CAD build for the part. Positions are in the model's coordinates, mm. Face numbers are marked on the shaded views. A direction names the side the tool comes from. Give positions to 0.01 mm unless a question says otherwise; leave off trailing zeros. Order: outer loops, then holes, each group sorted by start corner. A loop starts at its lowest first (then second) coordinate and runs counter-clockwise, first axis right, second up. Notation, with made-up numbers: (1.5, 12.5) -> (29.5, 12.5) arc R27 ccw to (29.5, 45.5) -> close; hole circle Ø8 at (50, 87.25). An arc over 180 degrees is marked (long way). Use one line per item in the form item = value. Start each with the question number.
1) Cut at B-B, the plane y = 15. Give the cut face in (x, z) (3 decimals), and give its area (3 significant figures).
2) Mould opens along Z. For the marked faces 4 and 5 say: pulls with the +Z half, pulls with the -Z half, needs draft (parallel to the pull), parting line crosses it, or undercut.
3) Cut at C-C, the plane z = -52. Give the cut face in (x, y) (3 decimals).
4) Cut at A-A, the plane x = 13.75. Give the cut face in (y, z) (3 decimals), and give its area (3 significant figures).
5) Drop flat-ended pins along their axis: P1, Ø12.5, axis at y = 14, z = -52, coming from the +X side; P2, Ø0.8, axis at x = 7, y = 41, coming from the +Z side (3 decimals); P3, Ø9, axis at y = -35, z = -30, coming from the +X side. Give the stop position or say it passes through.
6) Probe line 1 (Z direction, x = 6, y = 43) (3 decimals); line 2 (Z direction, x = 7.25, y = -13) (3 decimals); line 3 (Z direction, x = 6.5, y = -43) (3 decimals). List the from-to ranges inside material, lowest first.
7) Tool access for the marked faces 1, 2 and 3: list every direction of +Z, -Z, +X, -X, +Y, -Y with a clear straight run to the whole face (end or side of a thin tool).
8) Cut at D-D, the plane y = -39. Give the cut face in (x, z) (3 decimals).
from build123d import *

# Parameters (mm, degrees)
SKETCH1_W            = 100
SKETCH1_H            = 130
SKETCH1_W_2          = 32.89
SKETCH1_H_2          = 100.13
SKETCH1_R            = 1
BOSS_EXTRUDE1_DEPTH  = 5
SKETCH3_W            = 32.89
SKETCH3_H            = 100.13
SKETCH3_R            = 1
BOSS_EXTRUDE3_DEPTH  = 3
SKETCH4_W            = 16.6
SKETCH4_H            = 21.6
BOSS_EXTRUDE4_DEPTH  = 2.5
SKETCH5_W            = 60
SKETCH5_H            = 25
BOSS_EXTRUDE5_DEPTH  = 2.5
SKETCH6_W            = 18
SKETCH6_H            = 21
BOSS_EXTRUDE6_DEPTH  = 2
SKETCH7_W            = 8.4
SKETCH7_H            = 20
BOSS_EXTRUDE7_DEPTH  = 5
SKETCH9_W            = 2.5
SKETCH9_H            = 64.8
BOSS_EXTRUDE8_DEPTH  = 5
SKETCH10_W           = 23.22
SKETCH10_H           = 2.5
BOSS_EXTRUDE9_DEPTH  = 18.22
SKETCH12_W           = 26
SKETCH12_H           = 36
BOSS_EXTRUDE11_DEPTH = 5
SKETCH11_W           = 26
SKETCH11_H           = 36
BOSS_EXTRUDE10_DEPTH = 5


with BuildPart() as part:
    # Sketch1 → Boss-Extrude1 (new body)
    # profile 1 of 2: a face of its own
    with BuildSketch(Plane(origin=(0, 0, 0), x_dir=(0, 0, -1), z_dir=(1, 0, 0))):
        with Locations((32.555, -9.935)):
            Rectangle(SKETCH1_W, SKETCH1_H)
        Rectangle(SKETCH1_W_2, SKETCH1_H_2, mode=Mode.SUBTRACT)
    # profile 2 of 2: a face of its own
    with BuildSketch(Plane(origin=(0, 0, 0), x_dir=(0, 0, -1), z_dir=(1, 0, 0))):
        Rectangle(SKETCH1_W_2, SKETCH1_H_2)
        with Locations((-13.855, -47.705)):
            Circle(SKETCH1_R, mode=Mode.SUBTRACT)
        with Locations((13.855, -47.705)):
            Circle(SKETCH1_R, mode=Mode.SUBTRACT)
        with Locations((13.855, 47.395)):
            Circle(SKETCH1_R, mode=Mode.SUBTRACT)
        with Locations((-13.855, 47.395)):
            Circle(SKETCH1_R, mode=Mode.SUBTRACT)
    extrude(amount=BOSS_EXTRUDE1_DEPTH)

    # Sketch3 → Boss-Extrude3 (add)
    with BuildSketch(Plane(origin=(5, 0, 0), x_dir=(0, 0, -1), z_dir=(1, 0, 0))):
        Rectangle(SKETCH3_W, SKETCH3_H)
        with Locations((-13.855, 47.395)):
            Circle(SKETCH3_R, mode=Mode.SUBTRACT)
        with Locations((13.855, 47.395)):
            Circle(SKETCH3_R, mode=Mode.SUBTRACT)
        with Locations((13.855, -47.705)):
            Circle(SKETCH3_R, mode=Mode.SUBTRACT)
        with Locations((-13.855, -47.705)):
            Circle(SKETCH3_R, mode=Mode.SUBTRACT)
    extrude(amount=BOSS_EXTRUDE3_DEPTH)

    # Sketch4 → Boss-Extrude4 (add)
    with BuildSketch(Plane(origin=(5, 0, 0), x_dir=(0, 0, -1), z_dir=(1, 0, 0))):
        with Locations((27.245, 39.265)):
            Rectangle(SKETCH4_W, SKETCH4_H)
    extrude(amount=BOSS_EXTRUDE4_DEPTH)

    # Sketch5 → Boss-Extrude5 (add)
    with BuildSketch(Plane(origin=(5, 0, 0), x_dir=(0, 0, -1), z_dir=(1, 0, 0))):
        with Locations((48.445, 13.965)):
            Rectangle(SKETCH5_W, SKETCH5_H)
    extrude(amount=BOSS_EXTRUDE5_DEPTH)

    # Sketch6 → Boss-Extrude6 (add)
    with BuildSketch(Plane(origin=(5, 0, 0), x_dir=(0, 0, -1), z_dir=(1, 0, 0))):
        with Locations((47.260487744, 39.246233232)):
            Rectangle(SKETCH6_W, SKETCH6_H)
    extrude(amount=BOSS_EXTRUDE6_DEPTH)

    # Sketch7 → Boss-Extrude7 (add)
    with BuildSketch(Plane(origin=(5, 0, 0), x_dir=(0, 0, -1), z_dir=(1, 0, 0))):
        with Locations((62.460487744, 38.465)):
            Rectangle(SKETCH7_W, SKETCH7_H)
    extrude(amount=BOSS_EXTRUDE7_DEPTH)

    # Sketch9 → Boss-Extrude8 (add)
    with BuildSketch(Plane(origin=(5, 0, 0), x_dir=(0, 0, -1), z_dir=(1, 0, 0))):
        with Locations((20.195, -35.935)):
            Rectangle(SKETCH9_W, SKETCH9_H)
        with Locations((40.915, -35.935)):
            Rectangle(SKETCH9_W, SKETCH9_H)
    extrude(amount=BOSS_EXTRUDE8_DEPTH)

    # Sketch10 → Boss-Extrude9 (add)
    with BuildSketch(Plane(origin=(5, 0, 0), x_dir=(0, 0, -1), z_dir=(1, 0, 0))):
        with Locations((30.555, -69.585)):
            Rectangle(SKETCH10_W, SKETCH10_H)
        with Locations((30.555, -2.285)):
            Rectangle(SKETCH10_W, SKETCH10_H)
    extrude(amount=BOSS_EXTRUDE9_DEPTH)

    # Sketch12 → Boss-Extrude11 (add)
    with BuildSketch(Plane(origin=(5, 0, 0), x_dir=(0, 0, -1), z_dir=(1, 0, 0))):
        with Locations((57.665, -19.035)):
            Rectangle(SKETCH12_W, SKETCH12_H)
    extrude(amount=BOSS_EXTRUDE11_DEPTH)

    # Sketch11 → Boss-Extrude10 (add)
    with BuildSketch(Plane(origin=(5, 0, 0), x_dir=(0, 0, -1), z_dir=(1, 0, 0))):
        with Locations((57.665, -19.035)):
            Rectangle(SKETCH11_W, SKETCH11_H)
    extrude(amount=BOSS_EXTRUDE10_DEPTH)


solid = part.part
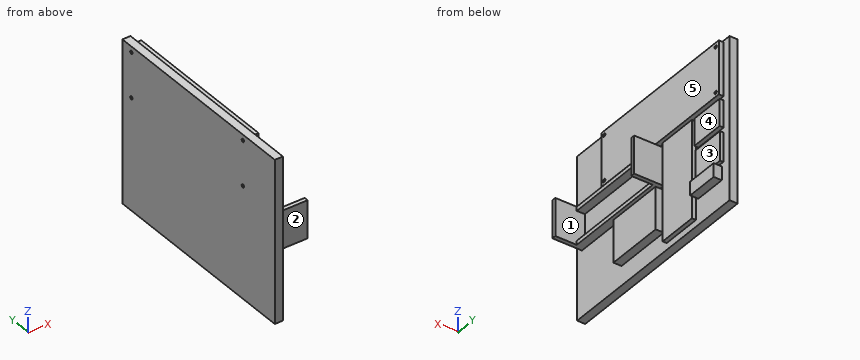
Result:
q1.outline = (0, -82.555) -> (5, -82.555) -> (5, -78.445) -> (7.5, -78.445) -> (7.5, -18.445) -> (5, -18.445) -> (5, -16.445) -> (8, -16.445) -> (8, 16.445) -> (5, 16.445) -> (5, 17.445) -> (0, 17.445) -> close
q1.area = 749 mm²
q2.face_4 = undercut
q2.face_5 = needs draft
q3.outline = (0, -74.935) -> (5, -74.935) -> (5, -37.035) -> (10, -37.035) -> (10, -1.035) -> (5, -1.035) -> (5, 1.465) -> (7.5, 1.465) -> (7.5, 26.465) -> (5, 26.465) -> (5, 28.746) -> (7, 28.746) -> (7, 49.746) -> (5, 49.746) -> (5, 55.065) -> (0, 55.065) -> close
q4.outline = (-70.835, -42.165) -> (-68.335, -42.165) -> (-68.335, -18.945) -> (-70.835, -18.945) -> close; (-3.535, -42.165) -> (-1.035, -42.165) -> (-1.035, -18.945) -> (-3.535, -18.945) -> close
q4.area = 116 mm²
q5.P1 = 7.5
q5.P2 = 16.445
q5.P3 = 5
q6.line_1 = -66.66 to -58.26, -56.26 to -38.26, -35.545 to -18.945, -16.445 to 16.445
q6.line_2 = -70.665 to -44.665, -42.165 to -39.665, -21.445 to -18.945, -16.445 to 16.445
q6.line_3 = -42.165 to -39.665, -21.445 to -18.945, -16.445 to 16.445
q7.face_1 = +X
q7.face_2 = +Z, -Z, +X, -Y
q7.face_3 = +X, +Y
q8.outline = (0, -82.555) -> (5, -82.555) -> (5, -42.165) -> (10, -42.165) -> (10, -39.665) -> (5, -39.665) -> (5, -21.445) -> (10, -21.445) -> (10, -18.945) -> (5, -18.945) -> (5, -16.445) -> (8, -16.445) -> (8, 16.445) -> (5, 16.445) -> (5, 17.445) -> (0, 17.445) -> close
